Part print with two shaded views. Sizes in mm from the minimum x, y, z corner. Give positions to 0.01 mm unless a question says otherwise; leave off trailing zeros. Write each loop counter-clockwise with the first axis right and the second up, starting at its lowest first coordinate (ties: lowest second). Pieces come first, ordered by that corner, then holes. Notation, with made-up numbers: M 8,-5.5 L 41,-5.5 A14 cw 41,21.5 Z; hole C -12.75,67 d7. An arc over 180 degrees is marked long. Return JSON: item names as keys, results as strings. Group by question number.
Q1. Band-saw the part on B-B, the plane z = 102. Give the cut face in (x, y).
Q2. Band-saw the part on A-A, the plane x = 560. Give the cut face in (y, z).
Q3. Wall check: probe 1 along Z at (x, y) = (125, 18.75); probe 2 along Z at (x, y) = (40, 16); probe 3 along X at (y, z) = (12.75, 87). Give the ranges that are in metal, low to high.
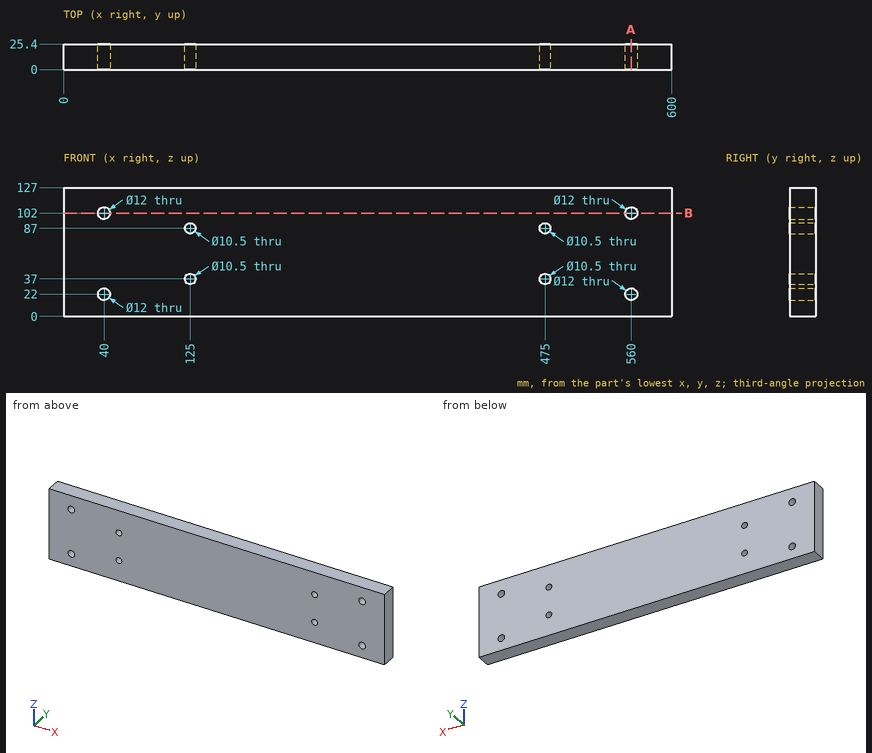
From the geometry:
{
 "1": {"outline": "M 0,0 L 34,0 L 34,25.4 L 0,25.4 Z; M 46,0 L 554,0 L 554,25.4 L 46,25.4 Z; M 566,0 L 600,0 L 600,25.4 L 566,25.4 Z"},
 "2": {"outline": "M 0,0 L 25.4,0 L 25.4,16 L 0,16 Z; M 0,28 L 25.4,28 L 25.4,96 L 0,96 Z; M 0,108 L 25.4,108 L 25.4,127 L 0,127 Z"},
 "3": {"probe 1": "z = 0 to 31.75, 42.25 to 81.75, 92.25 to 127", "probe 2": "z = 0 to 16, 28 to 96, 108 to 127", "probe 3": "x = 0 to 119.75, 130.25 to 469.75, 480.25 to 600"}
}
